Could you check a few things on this model? Use its own coordinates, in mm. A direction names the side the tool comes from. Coordinates: 2 decimals unless noted, no trailing zeros. Write each loop counter-clockwise with the first axis right and the second up, starting at its lowest first coordinate (ties: lowest second). Pieces come first, ordered by that corner, then holes. Notation, with made-up numbers: (-22.5, 27.5) - (20.5, 27.5) arc R9 ccw to (20.5, 34.5) - close; hole circle Ø7 at (43.25, 35.25). An arc over 180 degrees is marked (long way). Answer as a JSON object with one key per item and string values. Group by question number.
1) If we section it at D-D (y = 12): Write out the boundary of the cut face in (x, z), plus the area to 3 significant figures.
2) On a 3-axis mill with a long thin cutter (end or side, diameter ignored), from which of +Z, -Z, +X, -X, +Y, -Y can I reach the whole of each face in a straight line? I mean faces 1 (the flat face through (1, -6, 0)), 2 (the cylindrical face through (-7.91, -13.91, 1.48)), 3 (the flat face through (-33.5, 0, 1)). Say none if no direction works.
3) We'd pull the mould along Y, two halves only. Please class faces 4 (the flat face through (35, -5, 1)), 5 (the flat face through (36.5, -16, 1)): released by +Y, released by -Y, zero draft, split by the parting line, or undercut.
4) If we section it at C-C (z = 1.9): State how many separate pieces and enclosed holes the cut face has, plus the area to 3 significant figures.
5) If we section it at B-B (x = 27): Write out the boundary of the cut face in (y, z).
6) Please list where these lines run through material, in increasing order: line 1 along Y through (x, z) = (-12.5, 0.6); line 2 along X through (y, z) = (-1, 2.35); line 3 along Y through (x, z) = (3.5, 1.5).
7) If we section it at A-A (y = -3): Write out the boundary of the cut face in (x, z), plus the area to 3 significant figures.
8) Will these pins go through, and if not, where does the flat tip stop? pin 1 Ø8 at (x, y) = (22.5, -11) entering from -Z; pin 2 Ø0.9 at (y, z) = (27, 2) entering from -X; pin 3 Ø1.5 at (y, z) = (1.5, 1) entering from -X; pin 4 Ø0.9 at (x, z) = (2.5, 2) entering from -Y.
Autodesk Inventor part; units mm, degrees
ref_plane "YZ Plane" through (0, 0, 0) normal (1, 0, 0) x (0, 1, 0)
ref_plane "XZ Plane" through (0, 0, 0) normal (0, 1, 0) x (-1, 0, 0)
ref_plane "XY Plane" through (0, 0, 0) normal (0, 0, 1) x (1, 0, 0)
sketch "Sketch1" plane through (0, 0, 0) normal (0, 0, 1) x (1, 0, 0)
  line L0 (36.5, -28) -> (-36.5, -28)
  line L1 (-36.5, -28) -> (-36.5, 28)
  line L2 (-36.5, 28) -> (36.5, 28)
  line L3 (36.5, 28) -> (36.5, -28)
  line L4 (36.5, -28) -> (-36.5, 28) construction
  line L5 (-36.5, -28) -> (36.5, 28) construction
  point P0 (0, 0)
  dimension "d0" = 73
  dimension "d1" = 56
extrude "Extrusion1" add sketch "Sketch1" along normal blind 3
sketch "Sketch2" plane through (0, 0, 0) normal (0, 0, -1) x (-1, 0, 0)
  line L0 (36.5, -5) -> (33.5, -5)
  line L1 (33.5, -5) -> (33.5, 5)
  line L2 (33.5, 5) -> (36.5, 5)
  line L3 (36.5, 5) -> (36.5, -5)
  line L4 (36.5, -5) -> (33.5, 5) construction
  line L5 (33.5, -5) -> (36.5, 5) construction
  line L6 (36.5, 28) -> (36.5, -28)
  circle A0 centre (0, 0) radius 2
  circle A1 centre (0, 0) radius 8
  circle A2 centre (0, 0) radius 10.5
  circle A3 centre (0, 0) radius 16
  circle A4 centre (0, 0) radius 18.5
  line L7 (0, 0) -> (0, 10.5)
  line L8 (0, 0) -> (9.0933, 5.25)
  line L9 (0, 0) -> (0, 18.5)
  line L10 (0, 0) -> (-16.0215, 9.25)
  point P0 (35, 0)
  point P1 (36.5, 0)
  point P2 (-13.8564, 8)
  point P3 (0, 16)
  point P4 (6.9282, 4)
  point P5 (0, 8)
  dimension "d4" = 3
  dimension "d5" = 10
  dimension "d6" = 4
  dimension "d7" = 16
  dimension "d8" = 21
  dimension "d9" = 32
  dimension "d10" = 37
  dimension "d11" = 60
  dimension "d12" = 60
extrude "Extrusion3" cut sketch "Sketch2" against normal through all contours A0 L10 L8 | L8 L7 A0 | A0 L7 L10 | A1 L7 A2 L8 | L10 A4 L9 A3 picked at (-14.542, 9.8763)
fillet "Fillet1" radius 1 8 edges at (13.8564, 8, 1.5) (-6.9282, 4, 1.5) (0, 8, 1.5) (16.0215, 9.25, 1.5) (0, 10.5, 1.5) (-9.0933, 5.25, 1.5) (0, 16, 1.5) (0, 18.5, 1.5)
pattern_circular "Circular Pattern1" count 4 over 360 about axis through (0, 0, 0) along (0, 0, 1) of "Extrusion3", "Fillet1"
sketch "Sketch5" plane through (0, 0, 0) normal (0, 0, -1) x (-1, 0, 0)
  line L0 (5, 25) -> (-5, 25)
  line L1 (-5, 25) -> (-5, 28)
  line L2 (-5, 28) -> (5, 28)
  line L3 (5, 28) -> (5, 25)
  line L4 (5, 25) -> (-5, 28) construction
  line L5 (-5, 25) -> (5, 28) construction
  line L6 (36.5, 28) -> (36.5, -28)
  line L7 (-36.5, 28) -> (36.5, 28)
  line L8 (5, -28) -> (-5, -28)
  line L9 (-5, -28) -> (-5, -25)
  line L10 (-5, -25) -> (5, -25)
  line L11 (5, -25) -> (5, -28)
  line L12 (5, -28) -> (-5, -25) construction
  line L13 (-5, -28) -> (5, -25) construction
  line L14 (36.5, -28) -> (-36.5, -28)
  line L15 (-36.5, 5) -> (-33.5, 5)
  line L16 (-33.5, 5) -> (-33.5, -5)
  line L17 (-33.5, -5) -> (-36.5, -5)
  line L18 (-36.5, -5) -> (-36.5, 5)
  line L19 (-36.5, 5) -> (-33.5, -5) construction
  line L20 (-33.5, 5) -> (-36.5, -5) construction
  line L21 (-36.5, -28) -> (-36.5, 28)
  line L22 (33.5, 5) -> (36.5, 5)
  line L23 (36.5, 5) -> (36.5, -5)
  line L24 (36.5, -5) -> (33.5, -5)
  line L25 (33.5, -5) -> (33.5, 5)
  line L26 (33.5, 5) -> (36.5, -5) construction
  line L27 (36.5, 5) -> (33.5, -5) construction
  point P0 (0, 0)
  point P1 (0, 26.5)
  point P2 (0, 28)
  point P3 (0, -26.5)
  point P4 (0, -28)
  point P5 (-35, 0)
  point P6 (-36.5, 0)
  point P7 (35, 0)
  point P8 (36.5, 0)
  dimension "d31" = 10
  dimension "d32" = 3
  dimension "d33" = 36.5
  dimension "d34" = 10
  dimension "d35" = 3
  dimension "d36" = 3
  dimension "d37" = 10
  dimension "d38" = 3
  dimension "d39" = 10
extrude "Extrusion6" cut sketch "Sketch5" against normal through all contours L0 L1 L2 L3 | L6 L24 L25 L22 | L15 L16 L17 L18 | L8 L9 L10 L11
sketch "Sketch6" plane through (0, 0, 0) normal (0, 0, -1) x (-1, 0, 0)
  line L0 (-36.5, 28) -> (-5, 28)
  line L1 (5, 28) -> (36.5, 28)
  line L2 (5, 25) -> (-5, 25)
  line L3 (5, 28) -> (5, 25)
  line L4 (-5, 25) -> (-5, 28)
  line L5 (-5, 28) -> (5, 28)
  line L6 (-5, 25) -> (-36.5, 25)
  line L7 (-36.5, 5) -> (-36.5, 28)
  line L8 (5, 25) -> (36.5, 25)
  line L9 (36.5, 28) -> (36.5, 5)
  point P0 (0, 0)
extrude "Extrusion7" add sketch "Sketch6" against normal blind 3 contours L5 L3 L2 L4
extrude "Extrusion8" cut sketch "Sketch6" against normal through all contours L0 L4 L6 L7 | L1 L9 L8 L3
sketch "Sketch7" plane through (0, 0, 3) normal (0, 0, 1) x (1, 0, 0)
  line L0 (-5, -25) -> (-5, -28)
  line L1 (-5, -28) -> (-36.5, -28)
  line L2 (-36.5, -28) -> (-36.5, -5)
  line L3 (-36.5, -5) -> (-33.5, -5)
  line L4 (-33.5, -5) -> (-33.5, 5)
  line L5 (-33.5, 5) -> (-36.5, 5)
  line L6 (-36.5, 5) -> (-36.5, 25)
  line L7 (-36.5, 25) -> (-5, 25)
  line L8 (-5, 25) -> (-5, 28)
  line L9 (-5, 28) -> (5, 28)
  line L10 (5, 28) -> (5, 25)
  line L11 (5, 25) -> (36.5, 25)
  line L12 (36.5, 25) -> (36.5, 5)
  line L13 (36.5, 5) -> (33.5, 5)
  line L14 (33.5, 5) -> (33.5, -5)
  line L15 (33.5, -5) -> (36.5, -5)
  line L16 (36.5, -5) -> (36.5, -28)
  line L17 (36.5, -28) -> (5, -28)
  line L18 (5, -28) -> (5, -25)
  line L19 (5, -25) -> (-5, -25)
  arc A0 (16.9706, 0) -> (15.9723, -0.9412) centre (16.9706, -1) ccw
  arc A1 (8.8012, -13.3618) -> (15.9723, -0.9412) centre (0, 0) ccw
  arc A2 (8.8012, -13.3618) -> (8.4853, -14.6969) centre (9.3513, -14.1969) ccw
  line L20 (8.4853, -14.6969) -> (8.7357, -15.1307)
  arc A3 (8.7357, -15.1307) -> (10.1504, -15.4667) centre (9.6017, -14.6307) ccw
  arc A4 (10.1504, -15.4667) -> (18.4698, -1.0571) centre (0, 0) ccw
  arc A5 (18.4698, -1.0571) -> (17.4714, 0) centre (17.4714, -1) ccw
  line L21 (17.4714, 0) -> (16.9706, 0)
  arc A6 (6.178, 8.4901) -> (4.7236, 8.1815) centre (5.5896, 7.6815) ccw
  line L22 (4.7236, 8.1815) -> (4.4721, 7.746)
  arc A7 (4.4721, 7.746) -> (4.745, 6.4409) centre (5.3382, 7.246) ccw
  arc A8 (7.9505, 0.8889) -> (4.745, 6.4409) centre (0, 0) ccw
  arc A9 (7.9505, 0.8889) -> (8.9443, 0) centre (8.9443, 1) ccw
  line L23 (8.9443, 0) -> (9.4472, 0)
  arc A10 (9.4472, 0) -> (10.4417, 1.1053) centre (9.4472, 1) ccw
  arc A11 (10.4417, 1.1053) -> (6.178, 8.4901) centre (0, 0) ccw
  arc A12 (0, -16.9706) -> (-0.9412, -15.9723) centre (-1, -16.9706) ccw
  arc A13 (-13.3618, -8.8012) -> (-0.9412, -15.9723) centre (0, 0) ccw
  arc A14 (-13.3618, -8.8012) -> (-14.6969, -8.4853) centre (-14.1969, -9.3513) ccw
  line L24 (-14.6969, -8.4853) -> (-15.1307, -8.7357)
  arc A15 (-15.1307, -8.7357) -> (-15.4667, -10.1504) centre (-14.6307, -9.6017) ccw
  arc A16 (-15.4667, -10.1504) -> (-1.0571, -18.4698) centre (0, 0) ccw
  arc A17 (-1.0571, -18.4698) -> (0, -17.4714) centre (-1, -17.4714) ccw
  line L25 (0, -17.4714) -> (0, -16.9706)
  arc A18 (8.4901, -6.178) -> (8.1815, -4.7236) centre (7.6815, -5.5896) ccw
  line L26 (8.1815, -4.7236) -> (7.746, -4.4721)
  arc A19 (7.746, -4.4721) -> (6.4409, -4.745) centre (7.246, -5.3382) ccw
  arc A20 (0.8889, -7.9505) -> (6.4409, -4.745) centre (0, 0) ccw
  arc A21 (0.8889, -7.9505) -> (0, -8.9443) centre (1, -8.9443) ccw
  line L27 (0, -8.9443) -> (0, -9.4472)
  arc A22 (0, -9.4472) -> (1.1053, -10.4417) centre (1, -9.4472) ccw
  arc A23 (1.1053, -10.4417) -> (8.4901, -6.178) centre (0, 0) ccw
  arc A24 (-16.9706, 0) -> (-15.9723, 0.9412) centre (-16.9706, 1) ccw
  arc A25 (-8.8012, 13.3618) -> (-15.9723, 0.9412) centre (0, 0) ccw
  arc A26 (-8.8012, 13.3618) -> (-8.4853, 14.6969) centre (-9.3513, 14.1969) ccw
  line L28 (-8.4853, 14.6969) -> (-8.7357, 15.1307)
  arc A27 (-8.7357, 15.1307) -> (-10.1504, 15.4667) centre (-9.6017, 14.6307) ccw
  arc A28 (-10.1504, 15.4667) -> (-18.4698, 1.0571) centre (0, 0) ccw
  arc A29 (-18.4698, 1.0571) -> (-17.4714, 0) centre (-17.4714, 1) ccw
  line L29 (-17.4714, 0) -> (-16.9706, 0)
  arc A30 (-6.178, -8.4901) -> (-4.7236, -8.1815) centre (-5.5896, -7.6815) ccw
  line L30 (-4.7236, -8.1815) -> (-4.4721, -7.746)
  arc A31 (-4.4721, -7.746) -> (-4.745, -6.4409) centre (-5.3382, -7.246) ccw
  arc A32 (-7.9505, -0.8889) -> (-4.745, -6.4409) centre (0, 0) ccw
  arc A33 (-7.9505, -0.8889) -> (-8.9443, 0) centre (-8.9443, -1) ccw
  line L31 (-8.9443, 0) -> (-9.4472, 0)
  arc A34 (-9.4472, 0) -> (-10.4417, -1.1053) centre (-9.4472, -1) ccw
  arc A35 (-10.4417, -1.1053) -> (-6.178, -8.4901) centre (0, 0) ccw
  arc A36 (0, 16.9706) -> (0.9412, 15.9723) centre (1, 16.9706) ccw
  arc A37 (13.3618, 8.8012) -> (0.9412, 15.9723) centre (0, 0) ccw
  arc A38 (13.3618, 8.8012) -> (14.6969, 8.4853) centre (14.1969, 9.3513) ccw
  line L32 (14.6969, 8.4853) -> (15.1307, 8.7357)
  arc A39 (15.1307, 8.7357) -> (15.4667, 10.1504) centre (14.6307, 9.6017) ccw
  arc A40 (15.4667, 10.1504) -> (1.0571, 18.4698) centre (0, 0) ccw
  arc A41 (1.0571, 18.4698) -> (0, 17.4714) centre (1, 17.4714) ccw
  line L33 (0, 17.4714) -> (0, 16.9706)
  arc A42 (-8.4901, 6.178) -> (-8.1815, 4.7236) centre (-7.6815, 5.5896) ccw
  line L34 (-8.1815, 4.7236) -> (-7.746, 4.4721)
  arc A43 (-7.746, 4.4721) -> (-6.4409, 4.745) centre (-7.246, 5.3382) ccw
  arc A44 (-0.8889, 7.9505) -> (-6.4409, 4.745) centre (0, 0) ccw
  arc A45 (-0.8889, 7.9505) -> (0, 8.9443) centre (-1, 8.9443) ccw
  line L35 (0, 8.9443) -> (0, 9.4472)
  arc A46 (0, 9.4472) -> (-1.1053, 10.4417) centre (-1, 9.4472) ccw
  arc A47 (-1.1053, 10.4417) -> (-8.4901, 6.178) centre (0, 0) ccw
  circle A48 centre (0, 0) radius 2
properties part number "right"
Here are the results:
{
 "1": {"outline": "(-36.5, 0) - (-14.08, 0) - (-14.08, 3) - (-36.5, 3) - close; (-10.58, 0) - (10.58, 0) - (10.58, 3) - (-10.58, 3) - close; (14.08, 0) - (36.5, 0) - (36.5, 3) - (14.08, 3) - close", "area": "198 mm²"},
 "2": {"face 1": "-Z, +X, -X, +Y, -Y", "face 2": "+Z, -Z", "face 3": "+Z, -Z, -X"},
 "3": {"face 4": "undercut", "face 5": "zero draft"},
 "4": {"separate pieces": "1", "enclosed holes": "9", "area": "3,530 mm²"},
 "5": {"outline": "(-28, 0) - (25, 0) - (25, 3) - (-28, 3) - close"},
 "6": {"line 1": "y = -28 to -13.64, -9.99 to 9.99, 13.64 to 25", "line 2": "x = -33.5 to -10.45, -7.94 to -1.73, 1.73 to 15.97, 18.47 to 33.5", "line 3": "y = -25 to -9.9, -7.19 to 15.61, 18.17 to 28"},
 "7": {"outline": "(-33.5, 0) - (-10.06, 0) - (-10.06, 3) - (-33.5, 3) - close; (-7.42, 0) - (15.72, 0) - (15.72, 3) - (-7.42, 3) - close; (18.26, 0) - (33.5, 0) - (33.5, 3) - (18.26, 3) - close", "area": "185 mm²"},
 "8": {"pin 1": "stops at z = 0", "pin 2": "stops at x = -5", "pin 3": "stops at x = -33.5", "pin 4": "stops at y = -25"}
}
